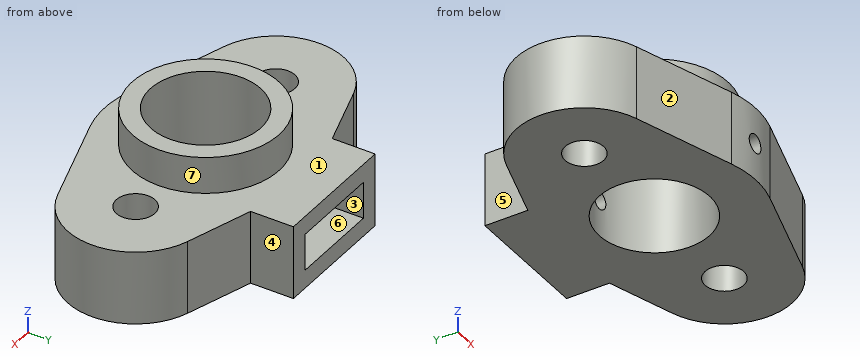
```python
from build123d import *

# Parameters (mm, degrees)
IZIM1_R                     = 10.5
IZIM1_R_2                   = 40
IZIM1_R_3                   = 30
Y_KSEKLIK_EKSTR_ZYON1_DEPTH = 20
IZIM3_R                     = 40
IZIM3_R_2                   = 30
Y_KSEKLIK_EKSTR_ZYON2_DEPTH = 20
IZIM4_W                     = 70
IZIM4_H                     = 40
Y_KSEKLIK_EKSTR_ZYON3_DEPTH = 40
IZIM6_W                     = 50
IZIM6_H                     = 20
KES_EKSTR_ZYON4_DEPTH       = 30
IZIM8_R                     = 5
KES_EKSTR_ZYON5_DEPTH       = 96


with BuildPart() as part:
    # Çizim1 → Yükseklik-Ekstrüzyon1 (new body, symmetric)
    with BuildSketch(Plane.XY):
        with BuildLine():
            Line((-71.077917778, -35.375500425), (-16.436310678, -52.48664298))
            ThreePointArc((-16.436310678, -52.48664298), (0, -55), (16.436310678, -52.48664298))
            Line((16.436310678, -52.48664298), (71.077917778, -35.375500425))
            ThreePointArc((71.077917778, -35.375500425), (97.06947926, 0), (71.077917778, 35.375500425))
            Line((71.077917778, 35.375500425), (16.436310678, 52.48664298))
            ThreePointArc((16.436310678, 52.48664298), (0, 55), (-16.436310678, 52.48664298))
            Line((-16.436310678, 52.48664298), (-71.077917778, 35.375500425))
            ThreePointArc((-71.077917778, 35.375500425), (-97.06947926, 0), (-71.077917778, -35.375500425))
        make_face()
        with Locations((-60, 0)):
            Circle(IZIM1_R, mode=Mode.SUBTRACT)
        with Locations((60, 0)):
            Circle(IZIM1_R, mode=Mode.SUBTRACT)
        Circle(IZIM1_R_2, mode=Mode.SUBTRACT)
        Circle(IZIM1_R_2)
        Circle(IZIM1_R_3, mode=Mode.SUBTRACT)
    extrude(amount=Y_KSEKLIK_EKSTR_ZYON1_DEPTH, both=True)

    # Çizim3 → Yükseklik-Ekstrüzyon2 (add)
    with BuildSketch(Plane.XY.offset(20)):
        Circle(IZIM3_R)
        Circle(IZIM3_R_2, mode=Mode.SUBTRACT)
    extrude(amount=Y_KSEKLIK_EKSTR_ZYON2_DEPTH)

    # Çizim4 → Yükseklik-Ekstrüzyon3 (add)
    with BuildSketch(Plane.XY.offset(20)):
        with Locations((0, 50)):
            Rectangle(IZIM4_W, IZIM4_H)
    extrude(amount=-Y_KSEKLIK_EKSTR_ZYON3_DEPTH)

    # Çizim6 → Kes-Ekstrüzyon4 (cut)
    with BuildSketch(Plane(origin=(0, 70, 0), x_dir=(1, 0, 0), z_dir=(0, 1, 0))):
        Rectangle(IZIM6_W, IZIM6_H)
    extrude(amount=-KES_EKSTR_ZYON4_DEPTH, mode=Mode.SUBTRACT)

    # Çizim8 → Kes-Ekstrüzyon5 (cut, through all)
    with BuildSketch(Plane(origin=(0, 40, 0), x_dir=(1, 0, 0), z_dir=(0, 1, 0))):
        Circle(IZIM8_R)
    extrude(amount=-KES_EKSTR_ZYON5_DEPTH, mode=Mode.SUBTRACT)


solid = part.part
```
Source: CAD feature listing. Evaluate the final solid. Frame: model axes, mm. Face numbers are marked on the shaded views. A direction names the side the tool comes from. Round coordinates to 2 decimals unless told otherwise and drop trailing zeros. Loops run counter-clockwise (first coordinate to the right, second up) from the corner with the lowest first, then second, coordinate; pieces in that order, holes last. Notation, with made-up numbers: M 11,25 L 20,25 A23 ccw 20,56 Z; hole C 78.5,-2.5 d6. An arc over 180 degrees is marked long. Use a Markdown table: item, result. Add a question column.
1. Reachability of the marked faces 4, 5, 6 and 7 from +Z, -Z, +X, -X, +Y, -Y: full face, straight path, thin tool, end or side. Return the list, or none.
2. Contact query for flat-ended pins moving along their axis: P1, Ø2, axis at x = -31, z = 12.5, coming from the -Y side; P2, Ø11.5, axis at x = 0, z = 0, coming from the +Y side; P3, Ø11.5, axis at y = 56, z = 2.5, coming from the +X side; P4, Ø6, axis at x = 0, z = 0, coming from the -Y side. Output: stop coordinate, or through.
3. Section query C-C on x = 0. Return the cut outline in (y, z).
4. Section query A-A on y = 0. Return the cut outline in (x, z).
5. Section query B-B on z = 0. Return the cut outline in (x, y), then the cut area to 3 significant figures.
6. Mould query, pull axis Z, two halves, no side actions, for the marked faces 1, 2 and 3. Classes: pulls with the +Z half, pulls with the -Z half, needs draft (parallel to the pull), parting line crosses it, or undercut.
7. Line query: line 1 (Z direction, x = 0, y = -48); line 2 (X direction, y = 62.5, z = 2.5); line 3 (Z direction, x = 70.5, y = -32). Output: solid intervals per line, ascending.
8. Section query D-D on y = 13.5. Return the cut outline in (x, z).
Reported:
| question | item | result |
|---|---|---|
| 1 | face 4 | +Z, -Z, +X, +Y |
| 1 | face 5 | +Z, -Z, -X, +Y |
| 1 | face 6 | +Y |
| 1 | face 7 | +Z |
| 2 | P1 | stops at y = -48.24 |
| 2 | P2 | stops at y = 40 |
| 2 | P3 | stops at x = 35 |
| 2 | P4 | passes through |
| 3 | outline | M -55,-20 L -30,-20 L -30,-5 L -55,-5 Z; M -55,5 L -30,5 L -30,40 L -40,40 L -40,20 L -55,20 Z; M 30,-20 L 70,-20 L 70,-10 L 40,-10 L 40,-5 L 30,-5 Z; M 30,5 L 40,5 L 40,10 L 70,10 L 70,20 L 40,20 L 40,40 L 30,40 Z |
| 4 | outline | M -97.07,-20 L -70.5,-20 L -70.5,20 L -97.07,20 Z; M -49.5,-20 L -30,-20 L -30,40 L -40,40 L -40,20 L -49.5,20 Z; M 30,-20 L 49.5,-20 L 49.5,20 L 40,20 L 40,40 L 30,40 Z; M 70.5,-20 L 97.07,-20 L 97.07,20 L 70.5,20 Z |
| 5 | outline | M -71.08,-35.38 L -16.44,-52.49 A55 ccw -5,-54.77 L -5,-29.58 A30 cw -5,29.58 L -5,40 L -25,40 L -25,70 L -35,70 L -35,46.67 L -71.08,35.38 A37.07 ccw Z; M 5,-54.77 A55 ccw 16.44,-52.49 L 71.08,-35.38 A37.07 ccw 71.08,35.38 L 35,46.67 L 35,70 L 25,70 L 25,40 L 5,40 L 5,29.58 A30 cw 5,-29.58 Z; hole C -60,0 d21; hole C 60,0 d21 |
| 5 | area | 11,800 mm² |
| 6 | face 1 | pulls with the +Z half |
| 6 | face 2 | needs draft |
| 6 | face 3 | undercut |
| 7 | line 1 | z = -20 to -5, 5 to 20 |
| 7 | line 2 | x = -35 to -25, 25 to 35 |
| 7 | line 3 | z = -20 to 20 |
| 8 | outline | M -94.52,-20 L -26.79,-20 L -26.79,40 L -37.65,40 L -37.65,20 L -94.52,20 Z; M 26.79,-20 L 94.52,-20 L 94.52,20 L 37.65,20 L 37.65,40 L 26.79,40 Z |
